The figure shows three views and two pictorial views of one solid part (mm, origin at its lowest corner). Answer the questions. A direction names the side the tool comes from. Give positions to 0.01 mm unless a question says otherwise; leave off trailing zeros. Order: outer loops, then holes, each group sorted by start corner. A loop starts at its lowest first (then second) coordinate and runs counter-clockwise, first axis right, second up. Notation, with made-up numbers: (-30, 6.5) -> (8, 6.5) arc R31 cw to (8, 34.5) -> close; hole circle Ø3 at (9, 57.5). An arc over 180 degrees is marked (long way). Use one line per item in the form item = value.
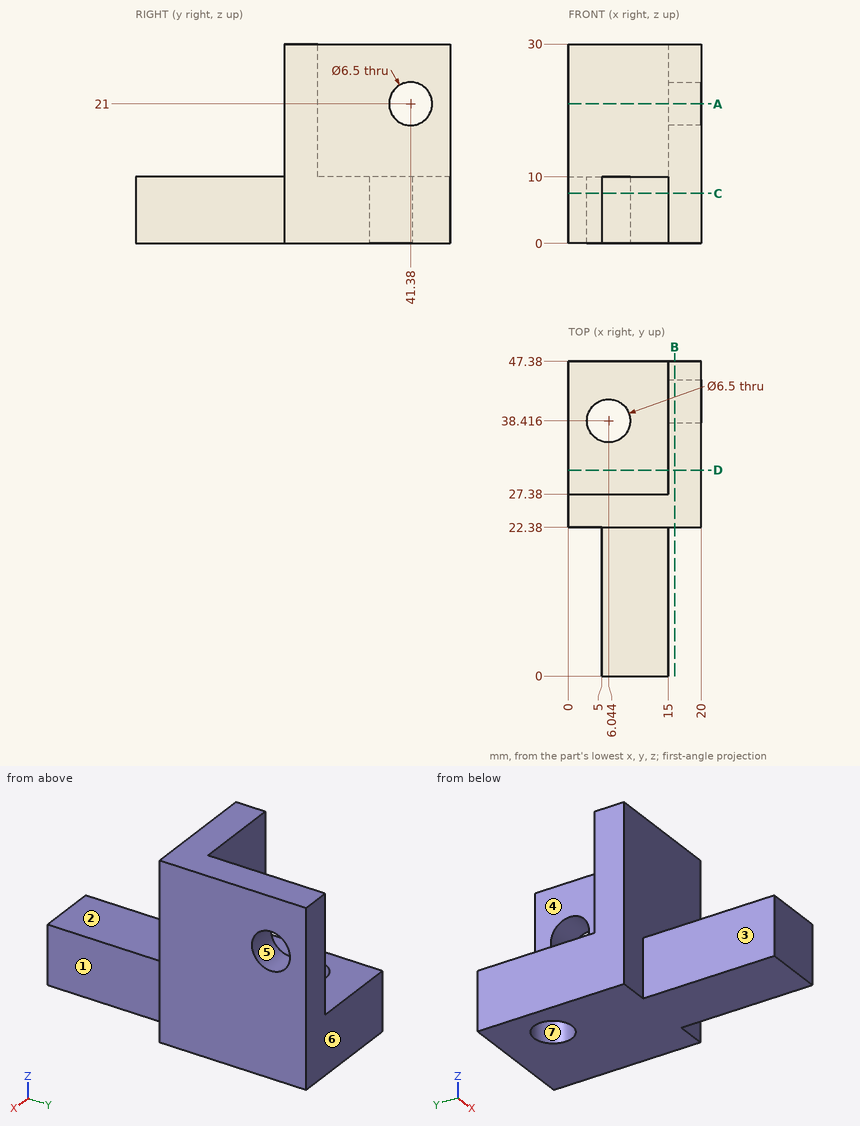
Item 1: Which of the six approach directions +Z, -Z, +X, -X, +Y, -Y give full straight-line access (tool end or side, diameter ignored) to the marked faces 1, 2 and 3?
Checks:
face_1 = +Z, -Z, +X, -Y
face_2 = +Z, +X, -X, -Y
face_3 = +Z, -Z, -X, -Y
Item 2: The part is cut by section C-C on z = 7.5. Give the vertices of the cut face in (x, y).
Checks:
outline = (0, 22.38) -> (5, 22.38) -> (5, 0) -> (15, 0) -> (15, 22.38) -> (20, 22.38) -> (20, 47.38) -> (0, 47.38) -> close; hole circle Ø6.5 at (6.04, 38.42)
Item 3: The part is cut by section D-D on y = 31. Give the vertices of the cut face in (x, z), and give its area (3 significant figures).
Checks:
outline = (0, 0) -> (20, 0) -> (20, 30) -> (15, 30) -> (15, 10) -> (0, 10) -> close
area = 300 mm²
Item 4: The part is cut by section B-B on x = 16. Give the vertices of the cut face in (y, z), and give its area (3 significant figures).
Checks:
outline = (22.38, 0) -> (47.38, 0) -> (47.38, 30) -> (22.38, 30) -> close; hole circle Ø6.5 at (41.38, 21)
area = 717 mm²
Item 5: Determine the mould class of the marked faces 4, 5, 6 and 7 for opening direction Y: +Y half, -Y half, draft (parallel to the pull), parting line (faces both ways), or undercut.
Checks:
face_4 = draft
face_5 = undercut
face_6 = +Y half
face_7 = undercut
Item 6: The part is cut by section A-A on z = 21. Give the vertices of the cut face in (x, y), and give its area (4 significant figures).
Checks:
outline = (0, 22.38) -> (20, 22.38) -> (20, 38.13) -> (15, 38.13) -> (15, 27.38) -> (0, 27.38) -> close; (15, 44.63) -> (20, 44.63) -> (20, 47.38) -> (15, 47.38) -> close
area = 167.5 mm²
Item 7: Given pin 1 Ø11 at (x, y) = (8, 10.5) entering from +Z; pin 2 Ø12 at (y, z) = (22.5, 25) entering from -X; pin 3 Ø3 at (y, z) = (6.5, 3) entering from +X; pin 4 Ø1 at (x, z) = (9, 24.5) entering from +Y, each flat-ended and moving along its own axis, determine where each tip first touches the part or whether it passes through.
Checks:
pin_1 = 10
pin_2 = 0
pin_3 = 15
pin_4 = 27.38
Item 8: Straight lines are drawn through the part: L1, parallel to Y at x = 18.6, z = 21; L2, parallel to Y at x = 14, z = 11.75; L3, parallel to Y at x = 17.75, z = 14. For each, find the intervals that lie inside material, in ascending order. Write a range as from..to.
Checks:
L1 = 22.38..38.13, 44.63..47.38
L2 = 22.38..27.38
L3 = 22.38..47.38
